Geometry: final body of the model. Coordinates: model frame, mm. A direction names the side the tool comes from. Coordinates: 2 decimals unless noted, no trailing zeros. Write each loop counter-clockwise with the first axis right and the second up, starting at its lowest first coordinate (ties: lowest second). Pieces come first, ordered by that corner, then holes. Notation, with made-up numbers: M 75,47.5 L 118,47.5 A30 cw 118,73.5 Z; hole C 49.25,13.5 d6. An arc over 180 degrees is marked long. Write item = value, one per line. Start each with the question number.
Item 1: Ray query, L1, parallel to X at y = 10.5, z = 15.5; L2, parallel to X at y = 6, z = 23; L3, parallel to Z at x = -36.5, y = 18. Return the intervals inside material, ascending. Write a range as [from, to].
Item 2: Section B-B on z = 6. Output: boundary loops of the cut face in (x, y).
Item 3: Reachability of faces 1 (the flat face through (-23.72, -7.89, 17.4)), 2 (the cylindrical face through (-48.12, 2.18, 4.93)), 3 (the cylindrical face through (39.084, 9.708, 17.395)), 4 (the flat face through (8, 24, 10)), 5 (the flat face through (33.897, -11.099, 17.395)) from +Z, -Z, +X, -X, +Y, -Y: full face, straight path, thin tool, end or side. Return the list, or none.
Item 4: Section A-A on x = -3. Output: boundary loops of the cut face in (y, z).
Item 5: Section D-D on x = 12.5. Output: boundary loops of the cut face in (y, z).
Item 6: Pull-direction query (Y, two-part tool) for faces 6 (the flat face through (0, 1, 0)), 7 (the cylindrical face through (12.518, -3.644, 12.325)), 8 (the cylindrical face through (-38.584, 5.187, 17.395)); classes: +Y half, -Y half, draft (parallel to the pull), parting line (faces both ways), or undercut.
Item 7: Section C-C on y = -19.5. Output: boundary loops of the cut face in (x, z), plus the area to 3 significant figures.
Item 8: First-contact query: pin 1 Ø5 at (x, y) = (-28.5, -22.5) entering from -Z; pin 2 Ø3 at (y, z) = (20.5, 20) entering from -X; pin 3 Ø8 at (y, z) = (-15, 10) entering from +X; pin 4 Ø19.5 at (x, y) = (14.34, 4.55) entering from +Z. Flat tips, straight axial feed; report the tip coordinate or a pass-through.
from build123d import *

# Parameters (mm, degrees)
F0_R     = 5.728623
F0_R_2   = 8.391993
F1_DEPTH = 25
F2_DEPTH = 10


with BuildPart() as f1:
    # F0 (on Top) → F1 (new body)
    with BuildSketch(Plane.XY):
        with BuildLine():
            Line((-12.392675, 28.53726), (-32.738149, 29.403025))
            Line((-32.738149, 29.403025), (-38.62714, 9.257409))
            ThreePointArc((-38.62714, 9.257409), (-38.565992, 5.131079), (-36.190918, 1.756265))
            Line((-36.190918, 1.756265), (-10.90472, -17.801028))
            Line((-10.90472, -17.801028), (28.572614, -26.104371))
            Line((28.572614, -26.104371), (39.37257, 4.333038))
            ThreePointArc((39.37257, 4.333038), (39.049502, 9.778257), (34.916635, 13.33834))
            Line((34.916635, 13.33834), (-12.392675, 28.53726))
        make_face()
        with BuildLine():
            ThreePointArc((6.730466, -6.065113), (-6.772657, -9.913719), (-16.715707, 0))
            Line((-16.715707, 0), (-12.846154, 1.013192))
            ThreePointArc((-12.846154, 1.013192), (-5.770901, -6.041189), (3.837619, -3.302607))
            Line((3.837619, -3.302607), (6.730466, -6.065113))
        make_face(mode=Mode.SUBTRACT)
        with Locations((-19.229598, 13.33834)):
            Circle(F0_R, mode=Mode.SUBTRACT)
        with Locations((14.337256, 4.548747)):
            Circle(F0_R_2, mode=Mode.SUBTRACT)
    extrude(amount=F1_DEPTH)

    # F0 (on Top) → F2 (join)
    with BuildSketch(Plane.XY):
        with BuildLine():
            Line((37.975333, 22.859074), (-10.619018, 38.470835))
            Line((-10.619018, 38.470835), (-33.34205, 39.437773))
            Line((-33.34205, 39.437773), (-42.405677, 31.972025))
            Line((-42.405677, 31.972025), (-48.22545, 12.063199))
            ThreePointArc((-48.22545, 12.063199), (-48.076948, 2.04211), (-42.30891, -6.153866))
            Line((-42.30891, -6.153866), (-15.208019, -27.114711))
            Line((-15.208019, -27.114711), (35.072481, -37.690305))
            Line((35.072481, -37.690305), (48.796888, 0.989053))
            ThreePointArc((48.796888, 0.989053), (48.012296, 14.213157), (37.975333, 22.859074))
        make_face()
        with BuildLine():
            Line((-38.62714, 9.257409), (-32.738149, 29.403025))
            Line((-32.738149, 29.403025), (-12.392675, 28.53726))
            Line((-12.392675, 28.53726), (34.916635, 13.33834))
            ThreePointArc((34.916635, 13.33834), (39.049502, 9.778257), (39.37257, 4.333038))
            Line((39.37257, 4.333038), (28.572614, -26.104371))
            Line((28.572614, -26.104371), (-10.90472, -17.801028))
            Line((-10.90472, -17.801028), (-36.190918, 1.756265))
            ThreePointArc((-36.190918, 1.756265), (-38.565992, 5.131079), (-38.62714, 9.257409))
        make_face(mode=Mode.SUBTRACT)
    extrude(amount=F2_DEPTH)


solid = f1.part
Responses:
q1.L1 = [-38.26, -24.21], [-14.25, 8.42], [20.25, 38.64]
q1.L2 = [-38.79, 6.07], [22.6, 39.74]
q1.L3 = [0, 10]
q2.outline = M -48.23,12.06 A17 ccw -42.31,-6.15 L -15.21,-27.11 L 35.07,-37.69 L 48.8,0.99 A17 ccw 37.98,22.86 L -10.62,38.47 L -33.34,39.44 L -42.41,31.97 Z; hole C -19.23,13.34 d11.46; hole M -16.72,0 A13.87 ccw 6.73,-6.07 L 3.84,-3.3 A9.87 cw -12.85,1.01 Z; hole C 14.34,4.55 d16.78
q3.face_1 = +Z, -X, -Y
q3.face_2 = +Z, -Z, -X
q3.face_3 = +Z, +X
q3.face_4 = +Z
q3.face_5 = +Z, +X, -Y
q4.outline = M -29.68,0 L -10.35,0 L -10.35,25 L -19.46,25 L -19.46,10 L -29.68,10 Z; M -6.35,0 L 36.02,0 L 36.02,10 L 25.52,10 L 25.52,25 L -6.35,25 Z
q5.outline = M -32.94,0 L -3.64,0 L -3.64,25 L -22.72,25 L -22.72,10 L -32.94,10 Z; M 12.74,0 L 31.04,0 L 31.04,10 L 20.54,10 L 20.54,25 L 12.74,25 Z
q6.face_6 = draft
q6.face_7 = undercut
q6.face_8 = parting line
q7.outline = M -25.05,0 L 41.53,0 L 41.53,10 L 30.92,10 L 30.92,25 L -2.83,25 L -2.83,10 L -25.05,10 Z
q7.area = 1,170 mm²
q8.pin_1 = through
q8.pin_2 = -35.78
q8.pin_3 = 44.54
q8.pin_4 = 25
